Can you work these out from the model? Positions are in its coordinate system, mm. A direction names the side the tool comes from. Coordinates: 2 decimals unless noted, no trailing zeros. Loops run counter-clockwise (first coordinate to the right, second up) from the corner with the lowest first, then second, coordinate; pieces in that order, holes last. Notation, with made-up numbers: M 68,21.5 L 112,21.5 A17 cw 112,54.5 Z; hole C 79.5,33.5 d10. An arc over 180 degrees is marked long. Answer as a JSON object with one key per item and string values. Group by question number.
Item 1: Which directions (+Z, -Z, +X, -X, +Y, -Y) give clear straight access to the entire face, cutting with the end or side of a thin tool? Please do faces 1 (the cylindrical face through (15.211, -68.327, 1.479)), 2 (the flat face through (28.232, -68.158, 1.479)).
Item 2: Suppose I cut it at D-D (y = -54). Write out the boundary of the cut face in (x, z).
Item 3: Suppose I cut it at C-C (z = 1.85). Write out the boundary of the cut face in (x, y), then the cut area to 3 significant figures.
Item 4: Suppose I cut it at A-A (y = -60). Write out the boundary of the cut face in (x, z), then the cut area to 3 significant figures.
Item 5: Suppose I cut it at B-B (x = 0). Write out the boundary of the cut face in (y, z), then the cut area to 3 significant figures.
Item 6: If I drill on line 1 (Y direction, x = 0, z = 1.3); line 2 (X direction, y = -40.5, z = 0.15); line 3 (Y direction, x = 16, z = 2), over which ranges is the centre line in solid material (lowest first)?
Item 7: We'd pull the mould along Y, two halves only. Please class faces 3 (the flat face through (3.512, -52, 1)), 4 (the cylindrical face through (0.806, -71.735, 1.521)), 5 (the cylindrical face through (0, -35, 2)), 6 (the cylindrical face through (-0.195, -58.513, 1.521)): +Y half, -Y half, draft (parallel to the pull), parting line (faces both ways), or undercut.
```python
from build123d import *

# Parameters (mm, degrees)
SKETCH_1_R          = 18
LASHENA_DEPTH       = 3
CUT_EXTRUDEA_DEPTH  = 3
WWW_KYTOOL_CN_COUNT = 16
SKETCH_3_R          = 1.5
CUT_EXTRUDE_2_DEPTH = 10
SKETCH_4_R          = 1.5
CUT_EXTRUDE_3_DEPTH = 10
SKETCH_5_W          = 7.023251592
SKETCH_5_H          = 5.670576874
EXTRUDE_3_DEPTH     = 3
SKETCH_6_R          = 1.5
CUT_EXTRUDE_4_DEPTH = 3
SKETCH_8_R          = 35
CUT_EXTRUDE_5_DEPTH = 3


with BuildPart() as part:
    # 草图1 → LaShenA (new body)
    with BuildSketch(Plane.XY):
        Circle(SKETCH_1_R)
    extrude(amount=LASHENA_DEPTH)

    # SketchA → Cut-ExtrudeA (cut)
    with BuildSketch(Plane.XY.offset(3)):
        with BuildLine():
            ThreePointArc((0.423212707, 13.493364703), (0, 13.5), (-0.423212707, 13.493364703))
            ThreePointArc((-0.423212707, 13.493364703), (-0.952770902, 13.685686791), (-1.20440395, 14.18977059))
            add(Edge.make_bspline(
                [(-1.20440395, 14.18977059), (-1.226562505, 14.455224305), (-1.213843633, 14.773889884), (-1.273675597, 15.110607864), (-1.299119688, 15.21139578), (-1.321432077, 15.29109757), (-1.349914152, 15.382250837), (-1.385146673, 15.484587535), (-1.427834192, 15.597770763), (-1.478623281, 15.721446817), (-1.538159915, 15.855229004), (-1.607069773, 15.998703507), (-1.685962928, 16.151428337), (-1.775430978, 16.312934487), (-1.876046532, 16.482726463), (-1.98836201, 16.660283053), (-2.112908684, 16.845058076), (-2.250195688, 17.036481179), (-2.400709063, 17.233958676), (-2.56491084, 17.43687441), (-2.743238138, 17.644590662), (-2.936102365, 17.856449073), (-3.14388814, 18.07177164), (-3.447378451, 18.368492697), (-3.689495989, 18.585006365), (-3.858042439, 18.727457792)],
                knots=[0.122308221, 0.122308221, 0.122308221, 0.122308221, 0.250610689, 0.276296194, 0.287604067, 0.300967916, 0.316387742, 0.333863545, 0.353395324, 0.37498308, 0.398626813, 0.424326522, 0.452082207, 0.48189387, 0.513761509, 0.547685125, 0.583664717, 0.621700286, 0.661791832, 0.703939355, 0.748142854, 0.79440233, 0.842717782, 0.893089212, 1, 1, 1, 1], degree=3))
            ThreePointArc((-3.858042439, 18.727457792), (0, 19.120726106), (3.858042439, 18.727457792))
            add(Edge.make_bspline(
                [(1.20440395, 14.18977059), (1.226562505, 14.455224305), (1.213843633, 14.773889884), (1.273675597, 15.110607864), (1.299119688, 15.21139578), (1.321432077, 15.29109757), (1.349914152, 15.382250837), (1.385146673, 15.484587535), (1.427834192, 15.597770763), (1.478623281, 15.721446817), (1.538159915, 15.855229004), (1.607069773, 15.998703507), (1.685962928, 16.151428337), (1.775430978, 16.312934487), (1.876046532, 16.482726463), (1.98836201, 16.660283053), (2.112908684, 16.845058076), (2.250195688, 17.036481179), (2.400709063, 17.233958676), (2.56491084, 17.43687441), (2.743238138, 17.644590662), (2.936102365, 17.856449073), (3.14388814, 18.07177164), (3.447378451, 18.368492697), (3.689495989, 18.585006365), (3.858042439, 18.727457792)],
                knots=[0.122308221, 0.122308221, 0.122308221, 0.122308221, 0.250610689, 0.276296194, 0.287604067, 0.300967916, 0.316387742, 0.333863545, 0.353395324, 0.37498308, 0.398626813, 0.424326522, 0.452082207, 0.48189387, 0.513761509, 0.547685125, 0.583664717, 0.621700286, 0.661791832, 0.703939355, 0.748142854, 0.79440233, 0.842717782, 0.893089212, 1, 1, 1, 1], degree=3))
            ThreePointArc((1.20440395, 14.18977059), (0.952770902, 13.685686791), (0.423212707, 13.493364703))
        make_face()
    cut_extrudea = extrude(amount=-CUT_EXTRUDEA_DEPTH, mode=Mode.SUBTRACT)

    # www.KYTool.cn: Cut-ExtrudeA ×16 about axis
    www_kytool_cn_axis = Axis((0, 0, -80.9), (0, 0, 1))
    for i in range(1, WWW_KYTOOL_CN_COUNT):
        add(cut_extrudea.rotate(www_kytool_cn_axis, i * 360 / WWW_KYTOOL_CN_COUNT), mode=Mode.SUBTRACT)

    # 草图3 → 切除-拉伸2 (cut)
    with BuildSketch(Plane(origin=(0, 0, 0), x_dir=(-1, 0, 0), z_dir=(0, 0, -1))):
        Circle(SKETCH_3_R)
    extrude(amount=-CUT_EXTRUDE_2_DEPTH, mode=Mode.SUBTRACT)

    # 草图4 → 切除-拉伸3 (cut)
    with BuildSketch(Plane(origin=(0, 0, 0), x_dir=(-1, 0, 0), z_dir=(0, 0, -1))):
        with Locations((5, 0)):
            Circle(SKETCH_4_R)
        with Locations((0, -5)):
            Circle(SKETCH_4_R)
        with Locations((-5, 0)):
            Circle(SKETCH_4_R)
        with Locations((0, 5)):
            Circle(SKETCH_4_R)
    extrude(amount=-CUT_EXTRUDE_3_DEPTH, mode=Mode.SUBTRACT)

    # 草图5 → 凸台-拉伸3 (add)
    with BuildSketch(Plane(origin=(0, 0, 0), x_dir=(-1, 0, 0), z_dir=(0, 0, -1))):
        with Locations((0, -14.81884661)):
            Rectangle(SKETCH_5_W, SKETCH_5_H)
        with BuildLine():
            ThreePointArc((3.511625796, -17.654135047), (0, -18), (-3.511625796, -17.654135047))
            Line((-3.511625796, -17.654135047), (-3.511625796, -69.911862257))
            ThreePointArc((-3.511625796, -69.911862257), (0, -70), (3.511625796, -69.911862257))
            Line((3.511625796, -69.911862257), (3.511625796, -17.654135047))
        make_face()
        with BuildLine():
            ThreePointArc((3.511625796, -69.911862257), (0, -70), (-3.511625796, -69.911862257))
            Line((-3.511625796, -69.911862257), (-3.511625796, -77.574694161))
            ThreePointArc((-3.511625796, -77.574694161), (0, -77.654135047), (3.511625796, -77.574694161))
            Line((3.511625796, -77.574694161), (3.511625796, -69.911862257))
        make_face()
        with BuildLine():
            Line((-3.511625796, -77.574694161), (-3.511625796, -69.911862257))
            ThreePointArc((-3.511625796, -69.911862257), (-15.374640932, -68.290705196), (-26.787840266, -64.671567276))
            Line((-26.787840266, -64.671567276), (-29.716950937, -71.743065985))
            ThreePointArc((-29.716950937, -71.743065985), (-16.868211219, -75.799921769), (-3.511625796, -77.574694161))
        make_face()
        with BuildLine():
            Line((3.511625796, -17.654135047), (-3.511625796, -17.654135047))
            ThreePointArc((-3.511625796, -17.654135047), (0, -18), (3.511625796, -17.654135047))
        make_face()
    extrude(amount=-EXTRUDE_3_DEPTH)

    # 草图6 → 切除-拉伸4 (cut)
    with BuildSketch(Plane.XY.offset(3)):
        with Locations((0, -60)):
            Circle(SKETCH_6_R)
        with Locations((0, -73)):
            Circle(SKETCH_6_R)
    extrude(amount=-CUT_EXTRUDE_4_DEPTH, mode=Mode.SUBTRACT)

    # 草图8 → 切除-拉伸5 (cut)
    with BuildSketch(Plane.XY.offset(3)):
        Circle(SKETCH_8_R)
    extrude(amount=-CUT_EXTRUDE_5_DEPTH, mode=Mode.SUBTRACT)


solid = part.part
```
From the geometry:
{
 "1": {"face 1": "+Z, -Z, +Y", "face 2": "+Z, -Z, +X, +Y"},
 "2": {"outline": "M -3.51,0 L 3.51,0 L 3.51,3 L -3.51,3 Z"},
 "3": {"outline": "M -3.51,-77.57 A77.65 ccw 29.72,-71.74 L 26.79,-64.67 A70 cw 3.51,-69.91 L 3.51,-34.82 A35 cw -3.51,-34.82 Z; hole C 0,-73 d3; hole C 0,-60 d3", "area": "481 mm2"},
 "4": {"outline": "M -3.51,0 L -1.5,0 L -1.5,3 L -3.51,3 Z; M 1.5,0 L 3.51,0 L 3.51,3 L 1.5,3 Z", "area": "12.1 mm2"},
 "5": {"outline": "M -77.65,0 L -74.5,0 L -74.5,3 L -77.65,3 Z; M -71.5,0 L -61.5,0 L -61.5,3 L -71.5,3 Z; M -58.5,0 L -35,0 L -35,3 L -58.5,3 Z", "area": "110 mm2"},
 "6": {"line 1": "-77.65 to -74.5, -71.5 to -61.5, -58.5 to -35", "line 2": "-3.51 to 3.51", "line 3": "-75.99 to -68.15"},
 "7": {"face 3": "draft", "face 4": "undercut", "face 5": "+Y half", "face 6": "undercut"}
}
